```python
from build123d import *

# Parameters (mm, degrees)
SKETCH_1_W      = 2
SKETCH_1_H      = 12.2
SKETCH_2_W      = 2
SKETCH_2_H      = 9
EXTRUDE_1_DEPTH = 17
FILLET_3_R      = 1


with BuildPart() as part:
    # 草图1 → 旋转1 (revolve)
    with BuildSketch(Plane(origin=(0, 0, 0), x_dir=(1, 0, 0), z_dir=(0, 1, 0))):
        with Locations((-1, -6.1)):
            Rectangle(SKETCH_1_W, SKETCH_1_H)
    revolve(axis=Axis((0, 0, 0), (-1, 0, 0)))

    # 草图2 → 凸台-拉伸1 (add)
    with BuildSketch(Plane.XY):
        with Locations((-1, 0)):
            Rectangle(SKETCH_2_W, SKETCH_2_H)
    extrude(amount=EXTRUDE_1_DEPTH)

    # 圆角3
    fillet_3_edges = [part.edges().sort_by_distance(p)[0] for p in [
        (-1, -4.5, 11.339753084),
        (-1, 4.5, 11.339753084),
    ]]
    fillet(fillet_3_edges, radius=FILLET_3_R)


solid = part.part
```
For this review, take the finished solid that the model builds, in its own axes (mm). A direction names the side the tool comes from. Coordinates: 2 decimals unless noted, no trailing zeros. Order: outer loops, then holes, each group sorted by start corner. A loop starts at its lowest first (then second) coordinate and runs counter-clockwise, first axis right, second up. Notation, with made-up numbers: (84.25, 80) - (130.25, 80) arc R18 ccw to (130.25, 88) - close; hole circle Ø10 at (-6.75, -16.5). An arc over 180 degrees is marked (long way). Answer as a JSON object with one key per item and string values. Group by question number.
1. Clearance check with flat-ended pins moving along their axes: P1, Ø1, axis at x = -1, z = 14.5, coming from the +Y side; P2, Ø1, axis at x = 0, z = 4.5, coming from the +Y side; P3, Ø0.6, axis at x = -1, z = 13.5, coming from the -Y side. State where each tip first meets the part, or that it passes through.
2. For probe 1 along Y at (x, z) = (-0.95, 0.25); probe 2 along Y at (x, z) = (-1.55, 14); probe 3 along Z at (x, y) = (-0.9, -2.5), list the stretches that pass through material, from the lowest coordinate up.
3. We need section A-A on y = -6.25. State the section outline as (x, z) points.
4. We need section B-B on z = 4.5. State the section outline as (x, y) points, then the cut area to 3 significant figures.
5. For faces 1 (the flat face through (-1, -4.5, 14)), 2 (the flat face through (-1, 0, 17)), 3 (the flat face through (-1, 4.5, 14)), list the 3-axis set-ups (+Z, -Z, +X, -X, +Y, -Y) from which the entire face can be reached by the end or side of a thin tool; tool diameter is ignored.
Final values:
{
 "1": {"P1": "y = 4.5", "P2": "y = 11.53", "P3": "y = -4.5"},
 "2": {"probe 1": "-12.2 to 12.2", "probe 2": "-4.5 to 4.5", "probe 3": "-11.94 to 17"},
 "3": {"outline": "(-2, -10.48) - (0, -10.48) - (0, 10.48) - (-2, 10.48) - close"},
 "4": {"outline": "(-2, -11.34) - (0, -11.34) - (0, 11.34) - (-2, 11.34) - close", "area": "45.4 mm²"},
 "5": {"face 1": "+Z, +X, -X, -Y", "face 2": "+Z, +X, -X, +Y, -Y", "face 3": "+Z, +X, -X, +Y"}
}
